from build123d import *

# Parameters (mm, degrees)
SKETCH_1_R          = 15
EXTRUDE_1_DEPTH     = 48
SKETCH_2_R          = 2
EXTRUDE_2_DEPTH     = 10
SKETCH_3_R          = 3
EXTRUDE_3_DEPTH     = 3
FILLET_1_R          = 1
FILLET_2_R          = 1
CUT_EXTRUDE_START   = 15
SKETCH_4_W          = 2
SKETCH_4_H          = 6
CUT_EXTRUDE_1_DEPTH = 3


with BuildPart() as part:
    # 草图1 → 凸台-拉伸1 (new body)
    with BuildSketch(Plane(origin=(0, 0, 0), x_dir=(0, 0, -1), z_dir=(1, 0, 0))):
        Circle(SKETCH_1_R)
    extrude(amount=-EXTRUDE_1_DEPTH)

    # 草图2 → 凸台-拉伸2 (add)
    with BuildSketch(Plane.ZY.offset(48)):
        with Locations(Location((0, 0, 0), (0, 0, 180))):
            Circle(SKETCH_2_R)
    extrude(amount=EXTRUDE_2_DEPTH)

    # 草图3 → 凸台-拉伸3 (add)
    with BuildSketch(Plane.ZY.offset(48)):
        with Locations(Location((0, 0, 0), (0, 0, 180))):
            Circle(SKETCH_3_R)
    extrude(amount=EXTRUDE_3_DEPTH)

    # 圆角1
    fillet_1_edges = [part.edges().sort_by_distance(p)[0] for p in [
        (-48, 0, 15),
    ]]
    fillet(fillet_1_edges, radius=FILLET_1_R)

    # 圆角2
    fillet_2_edges = [part.edges().sort_by_distance(p)[0] for p in [
        (0, 0, 15),
    ]]
    fillet(fillet_2_edges, radius=FILLET_2_R)

    # 草图4 → 切除-拉伸1 (cut)
    with BuildSketch(Plane(origin=(0, 0, 0), x_dir=(1, 0, 0), z_dir=(0, 1, 0)).offset(CUT_EXTRUDE_START)):
        with Locations((-2.5, 0.5)):
            Rectangle(SKETCH_4_W, SKETCH_4_H)
    extrude(amount=-CUT_EXTRUDE_1_DEPTH, mode=Mode.SUBTRACT)


solid = part.part
Can you work these out from the model? Positions are in its coordinate system, mm. A direction names the side the tool comes from. Coordinates: 2 decimals unless noted, no trailing zeros. Write each loop counter-clockwise with the first axis right and the second up, starting at its lowest first coordinate (ties: lowest second). Pieces come first, ordered by that corner, then holes. Notation, with made-up numbers: (21.5, 28.25) -> (39.5, 28.25) arc R24 cw to (39.5, 54.25) -> close; hole circle Ø5 at (48.5, 84.5). An arc over 180 degrees is marked (long way). Answer as CSV lines item,"result".
1) If I drill on line 1 (X direction, y = 1, z = 9.5); line 2 (Z direction, x = -36, y = 0.25); line 3 (Z direction, x = -7.5, y = -9), over which ranges is the centre line in solid material (lowest first)? Write a range as from..to.
Check result:
line 1,"-48..0"
line 2,"-15..15"
line 3,"-12..12"
2) If we mould it in two halves opening along X, with no side actions, what happens to faces 1 (the flat face through (-51, 1, -2)), 2 (the cylindrical face through (-49.48, -0.9, -2.86)), 3 (the flat face through (-3, 13, 2.5))? For each: +X half, -X half, draft (parallel to the pull), parting line (faces both ways), or undercut.
Check result:
face 1,"-X half"
face 2,"draft"
face 3,"undercut"
3) On a 3-axis mill with a long thin cutter (end or side, diameter ignored), from which of +Z, -Z, +X, -X, +Y, -Y can I reach the whole of each face in a straight line? I mean faces 4 (the flat face through (0, 0, 0)), 5 (the cylindrical face through (-54, 2, 0)), 6 (the flat face through (-3, 13, -3.5)). Say none if no direction works.
Check result:
face 4,"+Z, -Z, +X, +Y, -Y"
face 5,"-X"
face 6,"+Y"
4) If we section it at C-C on x = -15.5: Please give me the cut outline in (y, z), then the cut area to 3 significant figures.
Check result:
outline,"circle Ø30 at (0, 0)"
area,"707 mm²"
5) If we section it at A-A on z = 0: Please give me the cut outline in (x, y), then the cut area to 3 significant figures.
Check result:
outline,"(-58, -2) -> (-51, -2) -> (-51, -3) -> (-48, -3) -> (-48, -14) arc R1 ccw to (-47, -15) -> (-1, -15) arc R1 ccw to (0, -14) -> (0, 14) arc R1 ccw to (-1, 15) -> (-1.5, 15) -> (-1.5, 12) -> (-3.5, 12) -> (-3.5, 15) -> (-47, 15) arc R1 ccw to (-48, 14) -> (-48, 3) -> (-51, 3) -> (-51, 2) -> (-58, 2) -> close"
area,"1,480 mm²"
6) If we section it at B-B on y = 0: Please give me the cut outline in (x, z), then the cut area to 3 significant figures.
Check result:
outline,"(-58, -2) -> (-51, -2) -> (-51, -3) -> (-48, -3) -> (-48, -14) arc R1 ccw to (-47, -15) -> (-1, -15) arc R1 ccw to (0, -14) -> (0, 14) arc R1 ccw to (-1, 15) -> (-47, 15) arc R1 ccw to (-48, 14) -> (-48, 3) -> (-51, 3) -> (-51, 2) -> (-58, 2) -> close"
area,"1,490 mm²"
7) Will these pins go through, and if not, where does the flat tip stop? P1, Ø8, axis at x = -8.5, y = 5.5, coming from the +Z side; P2, Ø4, axis at y = -8.5, z = -7, coming from the -X side; P3, Ø0.6, axis at x = -2, y = 13.5, coming from the +Z side.
Check result:
P1,"z = 14.92"
P2,"x = -48"
P3,"z = 7.12"
